Verification items for the finished model (mm, model axes). A direction names the side the tool comes from. Round coordinates to 2 decimals unless told otherwise and drop trailing zeros. Loops run counter-clockwise (first coordinate to the right, second up) from the corner with the lowest first, then second, coordinate; pieces in that order, holes last. Notation, with made-up numbers: (11.25, 53) -> (60.25, 53) arc R22 cw to (60.25, 75) -> close; hole circle Ø7 at (31, 41). An arc over 180 degrees is marked (long way). Write item = value, one per line.
```python
from build123d import *

# Parameters (mm, degrees)
BOSS_EXTRUDE1_DEPTH     = 26
CUT_EXTRUDE1_DEPTH      = 106.834776893
CUT_EXTRUDE1_DEPTH_BACK = 106.834776893
SKETCH3_W               = 145
SKETCH3_H               = 23.5
CUT_EXTRUDE2_DEPTH      = 157.208194407
CUT_EXTRUDE2_DEPTH_BACK = 26
SKETCH4_W               = 65
SKETCH4_H               = 25


with BuildPart() as part:
    # Sketch2 → Boss-Extrude1 (new body)
    with BuildSketch(Plane(origin=(0, 0, 0), x_dir=(1, 0, 0), z_dir=(0, 1, 0))):
        with BuildLine():
            Line((-26.65, 70.5), (-26.65, 75))
            Line((-26.65, 75), (-35, 75))
            Line((-35, 75), (-35, -75))
            Line((-35, -75), (35, -75))
            Line((35, -75), (35, 75))
            Line((35, 75), (26.65, 75))
            Line((26.65, 75), (26.65, 70.5))
            Line((26.65, 70.5), (28.3, 70.5))
            ThreePointArc((28.3, 70.5), (25, 67.2), (21.7, 70.5))
            Line((21.7, 70.5), (23.35, 70.5))
            Line((23.35, 70.5), (23.35, 75))
            Line((23.35, 75), (-23.35, 75))
            Line((-23.35, 75), (-23.35, 70.5))
            Line((-23.35, 70.5), (-21.7, 70.5))
            ThreePointArc((-21.7, 70.5), (-25, 67.2), (-28.3, 70.5))
            Line((-28.3, 70.5), (-26.65, 70.5))
        make_face()
    extrude(amount=BOSS_EXTRUDE1_DEPTH)

    # Sketch3 → Cut-Extrude1 (cut, two sides: drawn at the far end of the back side and taken through both)
    with BuildSketch(Plane(origin=(35, 0, 0), x_dir=(0, 0, -1), z_dir=(1, 0, 0)).offset(-CUT_EXTRUDE1_DEPTH_BACK)):
        with Locations((0, 11.75)):
            Rectangle(SKETCH3_W, SKETCH3_H)
    extrude(amount=CUT_EXTRUDE1_DEPTH + CUT_EXTRUDE1_DEPTH_BACK, mode=Mode.SUBTRACT)

    # Sketch4 → Cut-Extrude2 (cut, two sides: drawn at the far end of the back side and taken through both)
    with BuildSketch(Plane.XY.offset(75).offset(-CUT_EXTRUDE2_DEPTH_BACK)):
        with Locations((0, 12.5)):
            Rectangle(SKETCH4_W, SKETCH4_H)
    extrude(amount=CUT_EXTRUDE2_DEPTH + CUT_EXTRUDE2_DEPTH_BACK, mode=Mode.SUBTRACT)


solid = part.part
```
(1) Sectioned sample at D-D, the plane x = 25. Record the cut outline in (y, z).
Filled sheet:
outline = (23.5, -67.2) -> (26, -67.2) -> (26, 75) -> (25, 75) -> (25, 49) -> (23.5, 49) -> close
(2) Sectioned sample at A-A, the plane y = 21.25. Record the cut outline in (x, z).
Filled sheet:
outline = (-35, -75) -> (-26.65, -75) -> (-26.65, -72.5) -> (-35, -72.5) -> close; (-35, 72.5) -> (-32.5, 72.5) -> (-32.5, 75) -> (-35, 75) -> close; (-23.35, -75) -> (23.35, -75) -> (23.35, -72.5) -> (-23.35, -72.5) -> close; (26.65, -75) -> (35, -75) -> (35, -72.5) -> (26.65, -72.5) -> close; (32.5, 72.5) -> (35, 72.5) -> (35, 75) -> (32.5, 75) -> close
(3) Sectioned sample at B-B, the plane x = -7.5. Record the cut outline in (y, z).
Filled sheet:
outline = (0, -75) -> (26, -75) -> (26, 75) -> (25, 75) -> (25, 49) -> (23.5, 49) -> (23.5, -72.5) -> (0, -72.5) -> close
(4) Go/stop test with flat-tipped pins: pin 1 Ø3 at (x, z) = (27.5, 39) entering from -Y; pin 2 Ø12.5 at (y, z) = (16, 60) entering from -X; pin 3 Ø12 at (x, y) = (8.5, 9) entering from +Z; pin 4 Ø0.8 at (x, y) = (14.5, 24) entering from +Z. Record where each tip stops, or that it passes through.
Filled sheet:
pin_1 = 23.5
pin_2 = through
pin_3 = -72.5
pin_4 = 49
(5) Draft check along X on faces 5 (the face through (-31, 13, -75)), 6 (the face through (-35, 24, -17)), 7 (the face through (-32.5, 17, 73)). Enter one of: released by +X, released by -X, zero draft, split by the parting line, or undercut.
Filled sheet:
face_5 = zero draft
face_6 = released by -X
face_7 = undercut
(6) Material ranges on probe 1 along Z at (x, y) = (10.5, 9); probe 2 along Y at (x, z) = (-12.5, -21); probe 3 along Y at (x, z) = (-12.5, 62), recorded low to high. Write a range as from..to.
Filled sheet:
probe_1 = -75..-72.5
probe_2 = 23.5..26
probe_3 = 25..26
(7) Sectioned sample at C-C, the plane z = -14.5. Record the cut outline in (x, y).
Filled sheet:
outline = (-35, 23.5) -> (35, 23.5) -> (35, 26) -> (-35, 26) -> close
(8) Set-up check for faces 1 (the face through (31, 12, -72.5)), 2 (the face through (23.35, 13, -74)), 3 (the face through (0, 25, 62)), 4 (the face through (0, 12, -72.5)): record each of +Z, -Z, +X, -X, +Y, -Y from which the full face is reachable in a straight line by a thin tool's end or side.
Filled sheet:
face_1 = +X, -X, -Y
face_2 = -Z, +Y, -Y
face_3 = +Z, -Y
face_4 = +Z, +X, -X, -Y
